Input: part model. Units: mm. Frame: model coordinates. A direction names the side the tool comes from. Give positions to 0.01 mm unless a question says otherwise; leave off trailing zeros. One line per question, with ' | ' between items.
from build123d import *

# Parameters (mm, degrees)
UPPER_AIRFRAME_COUPLER_SKETCH_R      = 43.15
UPPER_AIRFRAME_COUPLER_SKETCH_R_2    = 39.975
UPPER_AIRFRAME_COUPLER_EXTRUDE_DEPTH = 25
SHEAR_PIN_BORE_CUT_REACH             = 190.276
SHEAR_PIN_BORE_CUT_END_RADIUS        = 39.975
SHEAR_PIN_BORE_SKETCH_R              = 1.25
SHEAR_PIN_PATTERN_COUNT              = 4
CUT_EXTRUDE2_DEPTH                   = 40
CUT_EXTRUDE2_DEPTH_BACK              = 144.578301529
SKETCH1_R                            = 3


with BuildPart() as part:
    # Ellipsoid Sketch → Ellipsoid Revolve (revolve)
    with BuildSketch(Plane(origin=(0, 0, 0), x_dir=(0, 0, -1), z_dir=(1, 0, 0))):
        with BuildLine():
            Line((-150, 0), (-100, 0))
            add(Edge.make_bspline(
                [(0, 39.975), (-100, 39.975), (-100, 0)],
                knots=[4.71238898, 4.71238898, 4.71238898, 6.283185307, 6.283185307, 6.283185307], degree=2, weights=[1, 0.707106781, 1]))
            Line((0, 39.975), (0, 50))
            add(Edge.make_bspline(
                [(0, 50), (-150, 50), (-150, 0)],
                knots=[4.71238898, 4.71238898, 4.71238898, 6.283185307, 6.283185307, 6.283185307], degree=2, weights=[1, 0.707106781, 1]))
        make_face()
    revolve(axis=Axis((0, 0, -7.5), (0, 0, 1)))

    # Upper Airframe Coupler Sketch → Upper Airframe Coupler Extrude (add)
    with BuildSketch(Plane(origin=(0, 0, 0), x_dir=(-1, 0, 0), z_dir=(0, 0, -1))):
        Circle(UPPER_AIRFRAME_COUPLER_SKETCH_R)
        Circle(UPPER_AIRFRAME_COUPLER_SKETCH_R_2, mode=Mode.SUBTRACT)
    extrude(amount=UPPER_AIRFRAME_COUPLER_EXTRUDE_DEPTH)

    # Upper Airframe Mate Chamfer: read off the stored shape, not the designer's step
    # Upper Airframe Mate Chamfer outline → Upper Airframe Mate Chamfer (revolve, cut)
    with BuildSketch(Plane.XZ):
        Polygon((49.948616721, 6.798616721), (43.15, 0), (50, 0), (50, 6.798616721), align=None)
    revolve(axis=Axis((0, 0, 0), (0, 0, 1)), mode=Mode.SUBTRACT)

    # Shear Pin Bore Cut: up to this cylinder (the profile starts outside it)
    shear_pin_bore_cut_end = Plane(origin=(0, 0, -10), z_dir=(0, 0, -1)) * Cylinder(SHEAR_PIN_BORE_CUT_END_RADIUS, 461.502, mode=Mode.PRIVATE)
    # Shear Pin Bore Sketch → Shear Pin Bore Cut (cut, up to the surface)
    with BuildSketch(Plane(origin=(30.511657608, -30.511657608, 0), x_dir=(-0.7071067811865475, -0.7071067811865477, 0), z_dir=(0.7071067811865477, -0.7071067811865475, 0)), mode=Mode.PRIVATE) as shear_pin_bore_cut_sk1:
        with Locations(Location((0, 10, 0), (0, 0, 180))):
            Circle(SHEAR_PIN_BORE_SKETCH_R)
    shear_pin_bore_cut_tool1 = extrude(shear_pin_bore_cut_sk1.sketch, amount=-SHEAR_PIN_BORE_CUT_REACH, mode=Mode.PRIVATE) - shear_pin_bore_cut_end
    shear_pin_bore_cut = shear_pin_bore_cut_tool1.solids().sort_by_distance((30.511658, -30.511658, -10))[0]
    add(shear_pin_bore_cut, mode=Mode.SUBTRACT)

    # Shear Pin Pattern: Shear Pin Bore Cut ×4 about axis
    shear_pin_pattern_axis = Axis((0, 0, 0), (0, 0, 1))
    for i in range(1, SHEAR_PIN_PATTERN_COUNT):
        add(shear_pin_bore_cut.rotate(shear_pin_pattern_axis, i * 360 / SHEAR_PIN_PATTERN_COUNT), mode=Mode.SUBTRACT)

    # Sketch1 → Cut-Extrude2 (cut, two sides: drawn at the far end of the back side and taken through both)
    with BuildSketch(Plane.XY.offset(100).offset(-CUT_EXTRUDE2_DEPTH_BACK)):
        Circle(SKETCH1_R)
    extrude(amount=CUT_EXTRUDE2_DEPTH + CUT_EXTRUDE2_DEPTH_BACK, mode=Mode.SUBTRACT)


solid = part.part
1. Pin query (flat end, axial travel): P1, Ø1, axis at x = 35, y = -37, coming from the -Z side; P2, Ø10, axis at x = -21.5, y = 5, coming from the +Z side; P3, Ø1, axis at x = 24.5, z = 36, coming from the +Y side; P4, Ø5, axis at x = -29, y = -14.5, coming from the +Z side. Return the tip coordinate at first contact, or that it passes through.
Determined:
P1: passes through | P2: stops at z = 140.98 | P3: stops at y = 42.19 | P4: stops at z = 120.17
2. Reachability of faces 1 (the flat face through (0, 0, 140)), 2 (the cylindrical face through (-29.873, 28.923, -8.946)) from +Z, -Z, +X, -X, +Y, -Y: full face, straight path, thin tool, end or side. Return the list, or none.
Determined:
face 1: -Z | face 2: none
3. Ray query, line 1 along Y through (x, z) = (0, -16) (3 decimals); line 2 along X through (y, z) = (0, 125.5). Return the intervals inside material, ascending. Write a range as from..to.
Determined:
line 1: y = -43.15..-39.975, 39.975..43.15 | line 2: x = -27.39..-3, 3..27.39
4. Pull-direction query (X, two-part tool) for faces 3 (the cylindrical face through (-41.157, 12.961, -12.325)), 4 (the cylindrical face through (28.923, 29.873, -8.946)), 5 (the cylindrical face through (8.666, -39.024, -12.325)), 6 (the flat face through (-13, -38, -25)); classes: pulls with the +X half, pulls with the -X half, needs draft (parallel to the pull), parting line crosses it, or undercut.
Determined:
face 3: parting line crosses it | face 4: undercut | face 5: undercut | face 6: needs draft
